For this review, take the finished solid that the model builds, in its own axes (mm). A direction names the side the tool comes from. Coordinates: 2 decimals unless noted, no trailing zeros. Loops run counter-clockwise (first coordinate to the right, second up) from the corner with the lowest first, then second, coordinate; pieces in that order, holes last. Notation, with made-up numbers: (22, 33.25) -> (56, 33.25) arc R12 ccw to (56, 54.25) -> close; hole circle Ø9 at (-38.5, 89). An arc over 180 degrees is marked (long way). Answer in a Markdown table with one row per item.
from build123d import *

# Parameters (mm, degrees)
CROQUIS1_R              = 13.59
SALIENTE_EXTRUIR1_DEPTH = 45.34
CROQUIS2_R              = 4
SALIENTE_EXTRUIR2_DEPTH = 12.37
SALIENTE_EXTRUIR3_START = 12.37
CROQUIS3_R              = 4
SALIENTE_EXTRUIR3_DEPTH = 12.37
CROQUIS4_R              = 10.2
SALIENTE_EXTRUIR4_DEPTH = 14
CROQUIS5_R              = 9.44075635
SALIENTE_EXTRUIR5_DEPTH = 0.5
CROQUIS6_R              = 10.2
SALIENTE_EXTRUIR6_DEPTH = 4.5


with BuildPart() as part:
    # Croquis1 → Saliente-Extruir1 (new body)
    with BuildSketch(Plane(origin=(0, 0, 0), x_dir=(0, 0, -1), z_dir=(1, 0, 0))):
        with Locations(Location((0, 0, 0), (0, 0, 180))):
            Circle(CROQUIS1_R)
    extrude(amount=SALIENTE_EXTRUIR1_DEPTH)

    # Croquis2 → Saliente-Extruir2 (add)
    with BuildSketch(Plane(origin=(45.34, 0, 0), x_dir=(0, 0, -1), z_dir=(1, 0, 0))):
        Circle(CROQUIS2_R)
    extrude(amount=SALIENTE_EXTRUIR2_DEPTH)

    # Croquis3 → Saliente-Extruir3 (add)
    with BuildSketch(Plane.ZY.offset(SALIENTE_EXTRUIR3_START)):
        with Locations(Location((0, 0, 0), (0, 0, 180))):
            Circle(CROQUIS3_R)
    extrude(amount=-SALIENTE_EXTRUIR3_DEPTH)

    # Croquis4 → Saliente-Extruir4 (add)
    with BuildSketch(Plane(origin=(0, 0, 0), x_dir=(1, 0, 0), z_dir=(0, 1, 0))):
        with Locations(Location((30.34, 0, 0), (0, 0, 90))):
            Circle(CROQUIS4_R)
    extrude(amount=SALIENTE_EXTRUIR4_DEPTH)

    # Croquis5 → Saliente-Extruir5 (add)
    with BuildSketch(Plane(origin=(0, 14, 0), x_dir=(1, 0, 0), z_dir=(0, 1, 0))):
        with Locations(Location((30.34, 0, 0), (0, 0, 270))):
            Circle(CROQUIS5_R)
    extrude(amount=SALIENTE_EXTRUIR5_DEPTH)

    # Croquis6 → Saliente-Extruir6 (add)
    with BuildSketch(Plane(origin=(0, 14.5, 0), x_dir=(1, 0, 0), z_dir=(0, 1, 0))):
        with Locations(Location((30.34, 0, 0), (0, 0, 90))):
            Circle(CROQUIS6_R)
    extrude(amount=SALIENTE_EXTRUIR6_DEPTH)


solid = part.part
Item 1: Take a section at B-B, the plane x = 30.34. State the section outline as (y, z) points.
Worked answers:
| item | result |
|---|---|
| outline | (8.98, -10.2) -> (14, -10.2) -> (14, -9.44) -> (14.5, -9.44) -> (14.5, -10.2) -> (19, -10.2) -> (19, 10.2) -> (14.5, 10.2) -> (14.5, 9.44) -> (14, 9.44) -> (14, 10.2) -> (8.98, 10.2) arc R13.59 ccw (long way) to start |
Item 2: For L1, parallel to X at y = 10.5, z = -0.5; L2, parallel to Y at x = 28, z = -9.5; L3, parallel to Y at x = 8, z = 8.5, list the stretches that pass through material, from the lowest coordinate up.
Worked answers:
| item | result |
|---|---|
| L1 | 0 to 45.34 |
| L2 | -9.72 to 14, 14.5 to 19 |
| L3 | -10.6 to 10.6 |
Item 3: For faces 1 (the flat face through (0, 3, 3)), 2 (the flat face through (45.34, 3, 3)), 3 (the cylindrical face through (21.739, 16.718, -5.483)), 4 (the flat face through (37, 14.5, -7)), list the 3-axis set-ups (+Z, -Z, +X, -X, +Y, -Y) from which the entire face can be reached by the end or side of a thin tool; tool diameter is ignored.
Worked answers:
| item | result |
|---|---|
| face 1 | -X |
| face 2 | +X |
| face 3 | +Y |
| face 4 | none |
Item 4: Take a section at D-D, the plane x = -3.5. State the section outline as (y, z) points.
Worked answers:
| item | result |
|---|---|
| outline | circle Ø8 at (0, 0) |
Item 5: Insertion check: pin 1 (1.5 mm diameter, centred on y = -7.5, z = -2, fed in from +X); pin 2 (5 mm diameter, centred on y = 14.5, z = 3.5, fed in from -X); pin 3 (1 mm diameter, centred on x = 22.5, y = 10.5, fed in from +Z). Each pin has a flat end and moves straight along its axis. Give the tip position at first contact, or say it passes through.
Worked answers:
| item | result |
|---|---|
| pin 1 | x = 45.34 |
| pin 2 | x = 0 |
| pin 3 | z = 9.2 |
Item 6: Take a section at C-C, the plane z = 1.5. State the section outline as (x, y) points, and give its area (3 significant figures).
Worked answers:
| item | result |
|---|---|
| outline | (-12.37, -3.71) -> (0, -3.71) -> (0, -13.51) -> (45.34, -13.51) -> (45.34, -3.71) -> (57.71, -3.71) -> (57.71, 3.71) -> (45.34, 3.71) -> (45.34, 13.51) -> (40.43, 13.51) -> (40.43, 14) -> (39.66, 14) -> (39.66, 14.5) -> (40.43, 14.5) -> (40.43, 19) -> (20.25, 19) -> (20.25, 14.5) -> (21.02, 14.5) -> (21.02, 14) -> (20.25, 14) -> (20.25, 13.51) -> (0, 13.51) -> (0, 3.71) -> (-12.37, 3.71) -> close |
| area | 1,520 mm² |
Item 7: Take a section at A-A, the plane y = 0. State the section outline as (x, z) points, and give its area (3 significant figures).
Worked answers:
| item | result |
|---|---|
| outline | (-12.37, -4) -> (0, -4) -> (0, -13.59) -> (45.34, -13.59) -> (45.34, -4) -> (57.71, -4) -> (57.71, 4) -> (45.34, 4) -> (45.34, 13.59) -> (0, 13.59) -> (0, 4) -> (-12.37, 4) -> close |
| area | 1,430 mm² |
